Check sheet for the modelled part. Datum: model origin and axes. Units: mm. Give positions to 0.01 mm unless a question says otherwise; leave off trailing zeros. Loops run counter-clockwise (first coordinate to the right, second up) from the corner with the lowest first, then second, coordinate; pieces in that order, holes last. Notation, with made-up numbers: (63.5, -1) -> (108.5, -1) arc R9 cw to (108.5, 5) -> close; hole circle Ø8 at (-3, -29.75). An arc over 180 degrees is marked (long way). Answer as CSV lines item,"result". Start each with the question number.
(1) Material ranges on line 1 (Z direction, x = 0.45, y = -20) (3 decimals); line 2 (Y direction, x = 1.4, z = -43.34); line 3 (Y direction, x = 0.8, z = -37.5), recorded low to high. Write a range as from..to.
(2) Section check C-C on z = -43.34. Enter the section's corners in (x, y), plus the area to 3 significant figures.
(3) Section check B-B on x = 0.6. Enter the section's corners in (y, z) (3 decimals), plus the area to 3 significant figures.
(4) Section check A-A on y = -17.5. Enter the section's corners in (x, z) (3 decimals), plus the area to 3 significant figures.
Autodesk Inventor part; units mm, degrees
ref_plane "YZ Plane" through (0, 0, 0) normal (1, 0, 0) x (0, 1, 0)
ref_plane "XZ Plane" through (0, 0, 0) normal (0, 1, 0) x (-1, 0, 0)
ref_plane "XY Plane" through (0, 0, 0) normal (0, 0, 1) x (1, 0, 0)
sketch "Sketch1" plane through (0, 0, 0) normal (1, 0, 0) x (0, 1, 0)
  line L0 (0, 0) -> (-40, 0)
  line L1 (-40, 0) -> (-40, -66.53)
  line L2 (-40, -66.53) -> (0, -66.53)
  line L3 (0, -66.53) -> (0, 0)
  point P0 (-20, -33.265)
  dimension "d0" = 40
  dimension "d1" = 66.53
  dimension "d13" = 33.265
  dimension "d14" = 20
extrude "Extrusion1" add sketch "Sketch1" along normal blind 2.04
sketch "Sketch2" plane through (0, 0, 0) normal (1, 0, 0) x (0, 1, 0)
  line L0 (-26.55, -58.615) -> (-9.95, -58.615)
  line L1 (-9.95, -58.615) -> (-9.95, -50.815)
  line L2 (-9.95, -50.815) -> (-26.55, -50.815)
  line L3 (-26.55, -50.815) -> (-26.55, -58.615)
  line L4 (0, -66.53) -> (0, 0)
  line L5 (-40, -66.53) -> (0, -66.53)
  dimension "d4" = 16.6
  dimension "d5" = 7.8
  dimension "d11" = 9.95
  dimension "d12" = 7.915
extrude "Extrusion2" cut sketch "Sketch2" along normal mid plane 254
pattern_linear "Rectangular Pattern1" count 4 spacing 14.2 along (0, 0, 1) of "Extrusion2"
sketch "Sketch3" plane through (0, 0, 0) normal (1, 0, 0) x (0, 1, 0)
  circle A0 centre (-34.765, -51.34) radius 3.075
  line L0 (-40, -66.53) -> (0, -66.53)
  line L1 (-40, 0) -> (-40, -66.53)
  point P0 (0, 0)
  dimension "d15" = 6.15
  dimension "d16" = 15.19
  dimension "d17" = 5.235
extrude "Extrusion3" cut sketch "Sketch3" along normal up to next
pattern_linear "Rectangular Pattern2" count 2 spacing 8 along (0, 0, 1) of "Extrusion3"
sketch "Sketch4" plane through (0, 0, 0) normal (-1, 0, 0) x (0, 0, 1)
  circle A0 centre (-43.34, -34.765) radius 3.075
  circle A1 centre (-51.34, -34.765) radius 3.075
  line L0 (-8.215, -26.55) -> (-16.015, -26.55)
  line L1 (-16.015, -26.55) -> (-16.015, -9.95)
  line L2 (-16.015, -9.95) -> (-8.215, -9.95)
  line L3 (-8.215, -9.95) -> (-8.215, -26.55)
  line L4 (-22.415, -26.55) -> (-30.215, -26.55)
  line L5 (-30.215, -26.55) -> (-30.215, -9.95)
  line L6 (-30.215, -9.95) -> (-22.415, -9.95)
  line L7 (-22.415, -9.95) -> (-22.415, -26.55)
  line L8 (-36.615, -26.55) -> (-44.415, -26.55)
  line L9 (-44.415, -26.55) -> (-44.415, -9.95)
  line L10 (-44.415, -9.95) -> (-36.615, -9.95)
  line L11 (-36.615, -9.95) -> (-36.615, -26.55)
  line L12 (-50.815, -26.55) -> (-58.615, -26.55)
  line L13 (-58.615, -26.55) -> (-58.615, -9.95)
  line L14 (-58.615, -9.95) -> (-50.815, -9.95)
  line L15 (-50.815, -9.95) -> (-50.815, -26.55)
  line L16 (0, 0) -> (0, -40)
  line L17 (-66.53, 0) -> (0, 0)
  line L18 (-66.53, -40) -> (-66.53, 0)
  line L19 (0, -40) -> (-66.53, -40)
  circle A2 centre (-54.715, -13.85) radius 3.9
  circle A3 centre (-54.715, -22.65) radius 3.9
  circle A4 centre (-40.515, -13.85) radius 3.9
  circle A5 centre (-40.515, -22.65) radius 3.9
  circle A6 centre (-26.315, -13.85) radius 3.9
  circle A7 centre (-26.315, -22.65) radius 3.9
  circle A8 centre (-12.115, -13.85) radius 3.9
  circle A9 centre (-12.115, -22.65) radius 3.9
properties part number "temp_sensor_front_plate"
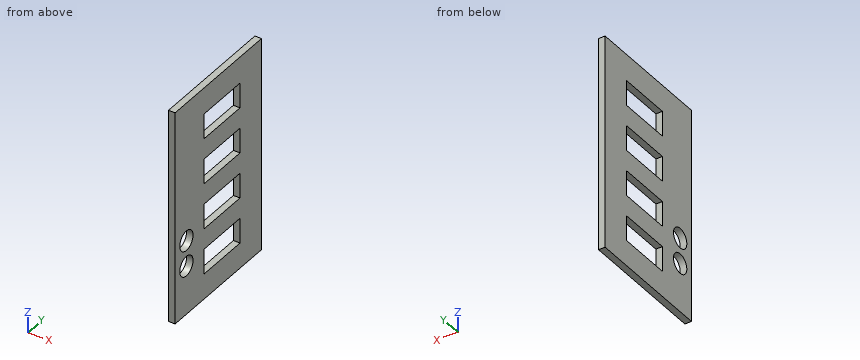
Working result:
1,line 1,"z = -66.53..-58.615, -50.815..-44.415, -36.615..-30.215, -22.415..-16.015, -8.215..0"
1,line 2,"y = -40..-37.84, -31.69..-26.55, -9.95..0"
1,line 3,"y = -40..-26.55, -9.95..0"
2,outline,"(0, -40) -> (2.04, -40) -> (2.04, -37.84) -> (0, -37.84) -> close; (0, -31.69) -> (2.04, -31.69) -> (2.04, -26.55) -> (0, -26.55) -> close; (0, -9.95) -> (2.04, -9.95) -> (2.04, 0) -> (0, 0) -> close"
2,area,"35.2 mm^2"
3,outline,"(-40, -66.53) -> (0, -66.53) -> (0, 0) -> (-40, 0) -> close; hole circle Ø6.15 at (-34.765, -51.34); hole circle Ø6.15 at (-34.765, -43.34); hole (-26.55, -58.615) -> (-9.95, -58.615) -> (-9.95, -50.815) -> (-26.55, -50.815) -> close; hole (-26.55, -44.415) -> (-9.95, -44.415) -> (-9.95, -36.615) -> (-26.55, -36.615) -> close; hole (-26.55, -30.215) -> (-9.95, -30.215) -> (-9.95, -22.415) -> (-26.55, -22.415) -> close; hole (-26.55, -16.015) -> (-9.95, -16.015) -> (-9.95, -8.215) -> (-26.55, -8.215) -> close"
3,area,"2,080 mm^2"
4,outline,"(0, -66.53) -> (2.04, -66.53) -> (2.04, -58.615) -> (0, -58.615) -> close; (0, -50.815) -> (2.04, -50.815) -> (2.04, -44.415) -> (0, -44.415) -> close; (0, -36.615) -> (2.04, -36.615) -> (2.04, -30.215) -> (0, -30.215) -> close; (0, -22.415) -> (2.04, -22.415) -> (2.04, -16.015) -> (0, -16.015) -> close; (0, -8.215) -> (2.04, -8.215) -> (2.04, 0) -> (0, 0) -> close"
4,area,"72.1 mm^2"
